```python
from build123d import *

# Parameters (mm, degrees)
SUSP_FR_LCA_FRONT_LEG_PROFILE_R         = 9.525
SUSP_FR_LCA_REAR_LEG_START              = 194.971257269
SUSP_FR_LCA_REAR_LEG_OUTLINE_R          = 9.525
SUSP_FR_LCA_REAR_LEG_DEPTH              = 392.368202981
SUSP_FR_LCA_REAR_LEG_START_2            = 587.33946025
SUSP_FR_LCA_REAR_LEG_2_OUTLINE_R        = 9.525
SUSP_FR_LCA_REAR_LEG_2_DEPTH            = 13.53250199
SUSP_FR_LCA_REAR_LEG_START_3            = 523.39106775
SUSP_FR_LCA_REAR_LEG_3_OUTLINE_W        = 26
SUSP_FR_LCA_REAR_LEG_3_OUTLINE_H        = 23
SUSP_FR_LCA_REAR_LEG_3_DEPTH            = 11.60893225
SUSP_FR_LCA_BUSH_FRONT_PROFILE_R        = 14
SUSP_FR_LCA_BUSH_REAR_PROFILE_R         = 14
SUSP_FR_PUSHROD_MOUNT_BRACKET_PROFILE_R = 8


with BuildPart() as part:
    # SUSP_FR_LCA_front_leg: sweep along a curve in space
    with BuildLine() as susp_fr_lca_front_leg_path:
        Line((205, -240.84, -42.383), (582, -130.461196, -55))
    # SUSP_FR_LCA_front_leg profile (on start of the path) → SUSP_FR_LCA_front_leg (sweep)
    with BuildSketch(Plane(origin=(205, -240.84, -42.383), x_dir=(-0.2809863080066093, 0.9597117768959672, 0), z_dir=(0.9592171404331008, 0.28084148736685866, -0.03210196992266429))):
        Circle(SUSP_FR_LCA_FRONT_LEG_PROFILE_R)
    sweep(path=susp_fr_lca_front_leg_path.line)

    # SUSP_FR_LCA_rear_leg: read off the stored shape, not the designer's step
    # SUSP_FR_LCA_rear_leg outline → SUSP_FR_LCA_rear_leg (add)
    with BuildSketch(Plane(origin=(0, 0, 0), x_dir=(0.3266773785489796, 0.9450726759891053, -0.01093286070332221), z_dir=(0.9445438654680327, -0.3268602715210149, -0.031610901725756396)).offset(SUSP_FR_LCA_REAR_LEG_START)):
        with Locations((67.432230038, -35.502420765)):
            Circle(SUSP_FR_LCA_REAR_LEG_OUTLINE_R)
    extrude(amount=SUSP_FR_LCA_REAR_LEG_DEPTH)

    # SUSP_FR_LCA_rear_leg 2 outline → SUSP_FR_LCA_rear_leg 2 (add)
    with BuildSketch(Plane(origin=(0, 0, 0), x_dir=(0.3266773785489796, 0.9450726759891053, -0.01093286070332221), z_dir=(0.9445438654680327, -0.3268602715210149, -0.031610901725756396)).offset(SUSP_FR_LCA_REAR_LEG_START_2)):
        with Locations((67.432230038, -35.502420765)):
            Circle(SUSP_FR_LCA_REAR_LEG_2_OUTLINE_R)
    extrude(amount=SUSP_FR_LCA_REAR_LEG_2_DEPTH)

    # SUSP_FR_LCA_rear_leg 3 outline → SUSP_FR_LCA_rear_leg 3 (cut)
    with BuildSketch(Plane(origin=(0, 0, 0), x_dir=(-0.28068434396715386, 0.959754165905817, 0.009393619012821172), z_dir=(0.9592171404331008, 0.2808414873668589, -0.03210196992266429)).offset(SUSP_FR_LCA_REAR_LEG_START_3)):
        with Locations((-289, -35.5)):
            Rectangle(SUSP_FR_LCA_REAR_LEG_3_OUTLINE_W, SUSP_FR_LCA_REAR_LEG_3_OUTLINE_H)
    extrude(amount=SUSP_FR_LCA_REAR_LEG_3_DEPTH, mode=Mode.SUBTRACT)

    # SUSP_FR_LCA_bush_front: sweep along a curve in space
    with BuildLine() as susp_fr_lca_bush_front_path:
        Line((205, -255.84, -42.383), (205, -225.84, -42.383))
    # SUSP_FR_LCA_bush_front profile (on start of the path) → SUSP_FR_LCA_bush_front (sweep)
    with BuildSketch(Plane(origin=(205, -255.84, -42.383), x_dir=(0, 0, 1), z_dir=(0, 1, 0))):
        Circle(SUSP_FR_LCA_BUSH_FRONT_PROFILE_R)
    sweep(path=susp_fr_lca_bush_front_path.line)

    # SUSP_FR_LCA_bush_rear: sweep along a curve in space
    with BuildLine() as susp_fr_lca_bush_rear_path:
        Line((205, -15, -42.383), (205, 15, -42.383))
    # SUSP_FR_LCA_bush_rear profile (on start of the path) → SUSP_FR_LCA_bush_rear (sweep)
    with BuildSketch(Plane(origin=(205, -15, -42.383), x_dir=(0, 0, 1), z_dir=(0, 1, 0))):
        Circle(SUSP_FR_LCA_BUSH_REAR_PROFILE_R)
    sweep(path=susp_fr_lca_bush_rear_path.line)

    # SUSP_FR_pushrod_mount_bracket: sweep along a curve in space
    with BuildLine() as susp_fr_pushrod_mount_bracket_path:
        Line((536.521845, -114.723439, -53.4779897), (535.6, -114.51, -83.23))
    # SUSP_FR_pushrod_mount_bracket profile (on start of the path) → SUSP_FR_pushrod_mount_bracket (sweep)
    with BuildSketch(Plane(origin=(536.521845, -114.723439, -53.4779897), x_dir=(-0.9995203321410445, 0, 0.0309694306802064), z_dir=(-0.030968634548961455, 0.007170309964793488, -0.999494637468947))):
        Circle(SUSP_FR_PUSHROD_MOUNT_BRACKET_PROFILE_R)
    sweep(path=susp_fr_pushrod_mount_bracket_path.line)


solid = part.part
```
Could you check a few things on this model? Use its own coordinates, in mm. A direction names the side the tool comes from. Give positions to 0.01 mm unless a question says otherwise; leave off trailing zeros. Order: outer loops, then holes, each group sorted by start corner. A loop starts at its lowest first (then second) coordinate and runs counter-clockwise, first axis right, second up.
Q1. If I drill on line 1 along Y through (x, z) = (233, -46.5); line 2 along Z through (x, y) = (222.5, -14); line 3 along Y through (x, z) = (526.5, -56), over which ranges is the centre line in solid material (lowest first)?
Q2. Suppose I cut it at A-A, the plane x = 205. Write out the boundary of the cut face in (y, z).
Q3. For faces 1 (the cylindrical face through (543.964, -114.245, -71.355)), 2 (the flat face through (205, -15, -43)), 3 (the flat face through (205, -255.84, -43)), which set-ups out of +Z, -Z, +X, -X, +Y, -Y let a thin tool reach every point of the face, with its end or its side?
Q4. I'm going to push flat-ended pins straight in: P1, Ø2, axis at x = 415.5, z = -55, coming from the -Y side; P2, Ø2, axis at x = 397, z = -43.5, coming from the -Y side; P3, Ø3, axis at x = 374, z = -54.5, coming from the -Y side. Where does each tip first touch, or does it pass through?
Q5. We'd pull the mould along Y, two halves only. Please class faces 4 (the flat face through (205, 15, -43)), 5 (the cylindrical face through (582.308, -140.645, -54.94)), 6 (the flat face through (205, -225.84, -43)): +Y half, -Y half, draft (parallel to the pull), parting line (faces both ways), or undercut.
Solution:
1. line 1: y = -241.97 to -223.26, -19.23 to -0.23
1. line 2: z = -48.92 to -37.19
1. line 3: y = -156.15 to -137.21, -120.9 to -101.67
2. outline: (-255.84, -56.38) - (-225.84, -56.38) - (-225.84, -28.38) - (-255.84, -28.38) - close; (-15, -56.38) - (15, -56.38) - (15, -28.38) - (-15, -28.38) - close
3. face 1: none
3. face 2: +Z, -Z, -X
3. face 3: +Z, -Z, +X, -X, -Y
4. P1: stops at y = -187.93
4. P2: stops at y = -193.6
4. P3: stops at y = -199.87
5. face 4: +Y half
5. face 5: -Y half
5. face 6: undercut
